```python
from build123d import *

# Parameters (mm, degrees)
SKETCH1_W           = 58
SKETCH1_H           = 15
SKETCH1_R           = 2
BOSS_EXTRUDE1_DEPTH = 5
FILLET1_R           = 5


with BuildPart() as part:
    # Sketch1 → Boss-Extrude1 (new body)
    with BuildSketch(Plane(origin=(0, 0, 0), x_dir=(1, 0, 0), z_dir=(0, 1, 0))):
        Rectangle(SKETCH1_W, SKETCH1_H)
        with Locations(Location((24, 0, 0), (0, 0, 270))):
            Circle(SKETCH1_R, mode=Mode.SUBTRACT)
        with Locations(Location((-24, 0, 0), (0, 0, 90))):
            Circle(SKETCH1_R, mode=Mode.SUBTRACT)
        with BuildLine():
            Line((1.9, -1.506859317), (-1.9, -1.506859317))
            ThreePointArc((-1.9, -1.506859317), (-2.425, 0), (-1.9, 1.506859317))
            Line((-1.9, 1.506859317), (1.9, 1.506859317))
            ThreePointArc((1.9, 1.506859317), (2.425, 0), (1.9, -1.506859317))
        make_face(mode=Mode.SUBTRACT)
    extrude(amount=BOSS_EXTRUDE1_DEPTH)

    # Fillet1
    fillet1_edges = [part.edges().sort_by_distance(p)[0] for p in [
        (29, 2.5, 7.5),
        (-29, 2.5, 7.5),
        (-29, 2.5, -7.5),
        (29, 2.5, -7.5),
    ]]
    fillet(fillet1_edges, radius=FILLET1_R)


solid = part.part
```
Source: CAD feature listing. Evaluate the final solid. Frame: model axes, mm. A direction names the side the tool comes from. Give positions to 0.01 mm unless a question says otherwise; leave off trailing zeros. Loops run counter-clockwise (first coordinate to the right, second up) from the corner with the lowest first, then second, coordinate; pieces in that order, holes last. Notation, with made-up numbers: (80.25, -20) - (113.25, -20) arc R6 ccw to (113.25, -9) - close; hole circle Ø8 at (22.5, 82.25). An arc over 180 degrees is marked (long way). Use CSV: the item, a comma, the result in double quotes. Start each with the question number.
1. Section C-C (z = 0). Output: boundary loops of the cut face in (x, y) (3 decimals).
2. Ray query, L1, parallel to Z at x = -24, y = 3.5; L2, parallel to X at y = 1.55, z = 0 (3 decimals); L3, parallel to X at y = 3.8, z = -1. Return the intervals inside material, ascending.
3. Section D-D (z = 6.5). Output: boundary loops of the cut face in (x, y).
4. Reachability of faces 5 (the flat face through (0, 5, -2)), 6 (the cylindrical face through (2.425, 2.465, -0.023)) from +Z, -Z, +X, -X, +Y, -Y: full face, straight path, thin tool, end or side. Return the list, or none.
5. Section A-A (x = 0). Output: boundary loops of the cut face in (y, z), then the cut area to 3 significant figures.
6. Draft query along Z for faces 1 (the cylindrical face through (-27.57, 2.54, 6)), 2 (the cylindrical face through (22.226, 2.465, 0.923)), 3 (the flat face through (-29, 2, 0)), 4 (the flat face through (0, 2, -7.5)). Return one class per face: +Z half, -Z half, draft (parallel to the pull), parting line (faces both ways), or undercut.
7. Section B-B (y = 1.9). Output: boundary loops of the cut face in (x, z) (3 decimals), then the cut area to 3 significant figures.
Response:
1,outline,"(-29, 0) - (-26, 0) - (-26, 5) - (-29, 5) - close; (-22, 0) - (-2.425, 0) - (-2.425, 5) - (-22, 5) - close; (2.425, 0) - (22, 0) - (22, 5) - (2.425, 5) - close; (26, 0) - (29, 0) - (29, 5) - (26, 5) - close"
2,L1,"-7.5 to -2, 2 to 7.5"
2,L2,"-29 to -26, -22 to -2.425, 2.425 to 22, 26 to 29"
2,L3,"-29 to -25.73, -22.27 to -2.21, 2.21 to 22.27, 25.73 to 29"
3,outline,"(-27, 0) - (27, 0) - (27, 5) - (-27, 5) - close"
4,face 5,"+Z, -Z, +X, -X, +Y"
4,face 6,"+Y, -Y"
5,outline,"(0, -7.5) - (5, -7.5) - (5, -1.51) - (0, -1.51) - close; (0, 1.51) - (5, 1.51) - (5, 7.5) - (0, 7.5) - close"
5,area,"59.9 mm²"
6,face 1,"+Z half"
6,face 2,"undercut"
6,face 3,"draft"
6,face 4,"-Z half"
7,outline,"(-29, -2.5) arc R5 ccw to (-24, -7.5) - (24, -7.5) arc R5 ccw to (29, -2.5) - (29, 2.5) arc R5 ccw to (24, 7.5) - (-24, 7.5) arc R5 ccw to (-29, 2.5) - close; hole circle Ø4 at (-24, 0); hole (-1.9, -1.507) - (1.9, -1.507) arc R2.425 ccw to (1.9, 1.507) - (-1.9, 1.507) arc R2.425 ccw to start; hole circle Ø4 at (24, 0)"
7,area,"810 mm²"
